CAD build for the part. Positions are in the model's coordinates, mm. A direction names the side the tool comes from. Give positions to 0.01 mm unless a question says otherwise; leave off trailing zeros. Write each loop counter-clockwise with the first axis right and the second up, starting at its lowest first coordinate (ties: lowest second). Pieces come first, ordered by that corner, then holes. Notation, with made-up numbers: (65, 12.5) - (85, 12.5) arc R22 cw to (85, 29.5) - close; hole circle Ø2 at (81.25, 88.5). An arc over 180 degrees is marked (long way). Answer as a JSON object with one key per item and string values.
from build123d import *
from build123d import SkipClean  # not in build123d's __all__

# Parameters (mm, degrees)
F1_DEPTH = 20
F0_W     = 2
F0_H     = 6.5
F5_DEPTH = 5
F6_DEPTH = 5


with BuildPart() as f1:
    # F0 (on Top) → F1 (new body, symmetric)
    with BuildSketch(Plane.XY):
        Polygon((-33.9359952807, -3.1263027601), (-33.9359952807, -23.1263027601), (-31.9359952807, -23.1263027601), (-32.4359952807, -6.1263027601), (-25.8359952807, -6.1263027601), (-25.8359952807, -23.1263027601), (-22.8359952807, -23.1263027601), (-17.8684814229, -20.8465269788), (-17.8684814229, -20.3465269788), (-17.8684814229, -13.8465269788), (-17.8684814229, -7.3465269788), (-17.8684814229, -6.8465269788), (-21.8359952807, -3.1263027601), align=None)
    extrude(amount=F1_DEPTH, both=True)

    # F0 (on Top) → F2 (revolve)
    with BuildSketch(Plane.XY):
        with Locations((-16.8684814229, -10.5965269788)):
            Rectangle(F0_W, F0_H)
    revolve(axis=Axis((-16.8684814229, -13.8465269788, 0), (1, 0, 0)))

    # F0 (on Top) → F3 (revolve)
    with BuildSketch(Plane.XY):
        Polygon((-9.0739962115, -8.8465269788), (-15.8684814229, -7.3465269788), (-15.8684814229, -13.8465269788), (-9.0739962115, -13.8465269788), align=None)
    revolve(axis=Axis((-4.8684814229, -13.8465269788, 0), (1, 0, 0)))

    # F0 (on Top) → F4 (revolve)
    with BuildSketch(Plane.XY):
        with BuildLine():
            Line((6.1315185771, -8.8465269788), (-9.0739962115, -8.8465269788))
            Line((-9.0739962115, -8.8465269788), (-9.0739962115, -13.8465269788))
            Line((-9.0739962115, -13.8465269788), (1.1315185771, -13.8465269788))
            ThreePointArc((1.1315185771, -13.8465269788), (2.5959846712, -10.3109930728), (6.1315185771, -8.8465269788))
        make_face()
        with BuildLine():
            Line((6.1315185771, -12.0965269788), (6.1315185771, -8.8465269788))
            ThreePointArc((6.1315185771, -8.8465269788), (2.5959846712, -10.3109930728), (1.1315185771, -13.8465269788))
            Line((1.1315185771, -13.8465269788), (4.3815185771, -13.8465269788))
            ThreePointArc((4.3815185771, -13.8465269788), (4.89408171, -12.6090901117), (6.1315185771, -12.0965269788))
        make_face()
        with BuildLine():
            Line((6.1315185771, -13.8465269788), (6.1315185771, -12.0965269788))
            ThreePointArc((6.1315185771, -12.0965269788), (4.89408171, -12.6090901117), (4.3815185771, -13.8465269788))
            Line((4.3815185771, -13.8465269788), (6.1315185771, -13.8465269788))
        make_face()
    revolve(axis=Axis((-4.8684814229, -13.8465269788, 0), (1, 0, 0)))

    # F0 (on Top) → F5 (cut, symmetric)
    with BuildSketch(Plane.XY):
        with BuildLine():
            Line((6.1315185771, -13.8465269788), (4.3815185771, -13.8465269788))
            ThreePointArc((4.3815185771, -13.8465269788), (4.89408171, -15.0839638459), (6.1315185771, -15.5965269788))
            Line((6.1315185771, -15.5965269788), (6.1315185771, -13.8465269788))
        make_face()
        with BuildLine():
            ThreePointArc((7.8815185771, -13.8465269788), (7.3689554442, -12.6090901117), (6.1315185771, -12.0965269788))
            Line((6.1315185771, -12.0965269788), (6.1315185771, -13.8465269788))
            Line((6.1315185771, -13.8465269788), (6.1315185771, -15.5965269788))
            ThreePointArc((6.1315185771, -15.5965269788), (7.3689554442, -15.0839638459), (7.8815185771, -13.8465269788))
        make_face()
        with BuildLine():
            Line((6.1315185771, -13.8465269788), (6.1315185771, -12.0965269788))
            ThreePointArc((6.1315185771, -12.0965269788), (4.89408171, -12.6090901117), (4.3815185771, -13.8465269788))
            Line((4.3815185771, -13.8465269788), (6.1315185771, -13.8465269788))
        make_face()
    extrude(amount=F5_DEPTH, both=True, mode=Mode.SUBTRACT)

    # F0 (on Top) → F6 (join, symmetric)
    with BuildSketch(Plane.XY):
        with BuildLine():
            Line((6.1315185771, -12.0965269788), (6.1315185771, -8.8465269788))
            ThreePointArc((6.1315185771, -8.8465269788), (2.5959846712, -10.3109930728), (1.1315185771, -13.8465269788))
            Line((1.1315185771, -13.8465269788), (4.3815185771, -13.8465269788))
            ThreePointArc((4.3815185771, -13.8465269788), (4.89408171, -12.6090901117), (6.1315185771, -12.0965269788))
        make_face()
        with BuildLine():
            Line((4.3815185771, -13.8465269788), (1.1315185771, -13.8465269788))
            ThreePointArc((1.1315185771, -13.8465269788), (2.5959846712, -17.3820608847), (6.1315185771, -18.8465269788))
            Line((6.1315185771, -18.8465269788), (6.1315185771, -15.5965269788))
            ThreePointArc((6.1315185771, -15.5965269788), (4.89408171, -15.0839638459), (4.3815185771, -13.8465269788))
        make_face()
        with BuildLine():
            ThreePointArc((11.1315185771, -13.8465269788), (9.667052483, -10.3109930728), (6.1315185771, -8.8465269788))
            Line((6.1315185771, -8.8465269788), (6.1315185771, -12.0965269788))
            ThreePointArc((6.1315185771, -12.0965269788), (7.3689554442, -12.6090901117), (7.8815185771, -13.8465269788))
            ThreePointArc((7.8815185771, -13.8465269788), (7.3689554442, -15.0839638459), (6.1315185771, -15.5965269788))
            Line((6.1315185771, -15.5965269788), (6.1315185771, -18.8465269788))
            ThreePointArc((6.1315185771, -18.8465269788), (9.667052483, -17.3820608847), (11.1315185771, -13.8465269788))
        make_face()
    with SkipClean():  # cleaning this boolean's faces spoils the solid; the shape is the same uncleaned
        extrude(amount=F6_DEPTH, both=True)


solid = f1.part
Item 1: Probe line 1 (X direction, y = -14, z = -0.5); line 2 (Y direction, x = -26, z = -8); line 3 (X direction, y = -19.25, z = 12). List the from-to ranges inside material, lowest first. Write a range as from..to.
Entries:
{"line 1": "-33.94..-32.2, -25.84..4.39, 7.87..11.13", "line 2": "-6.13..-3.13", "line 3": "-33.94..-32.05, -25.84..-17.87"}
Item 2: Which spindle directions (+Z, -Z, +X, -X, +Y, -Y) get a long thin tool onto all of the face, cutting with end or side? Do faces 1 (the flat face through (-25.836, -15, 0)), 2 (the flat face through (8.3, -13.8, 5)), 3 (the cylindrical face through (-3.267, -14.497, 4.957)), 4 (the flat face through (8.3, -13.8, -5)). Say none if no direction does.
Entries:
{"face 1": "+Z, -Z, -Y", "face 2": "+Z, +X, +Y, -Y", "face 3": "none", "face 4": "-Z, +X, +Y, -Y"}
Item 3: Flat gauge pins, fed straight in: P1, Ø4, axis at y = -15.5, z = -6.5, coming from the +X side; P2, Ø3, axis at y = -20.5, z = 7.5, coming from the +X side; P3, Ø3, axis at x = -2.5, y = -17.5, coming from the +Z side. Where does each tip first touch, or does it go through?
Entries:
{"P1": "x = 11.12", "P2": "x = -17.87", "P3": "z = 4.51"}
Item 4: Cut at C-C (y = -14.5). State how many separate pieces and enclosed holes the cut face has, and give its area (3 significant figures).
Entries:
{"separate pieces": "3", "enclosed holes": "0", "area": "660 mm2"}
Item 5: Cut at D-D (x = -20.5). Give the cut face in (y, z).
Entries:
{"outline": "(-22.05, -20) - (-4.38, -20) - (-4.38, 20) - (-22.05, 20) - close"}
Item 6: Cut at A-A (z = -11.5). Give the cut face in (x, y).
Entries:
{"outline": "(-33.94, -23.13) - (-31.94, -23.13) - (-32.44, -6.13) - (-25.84, -6.13) - (-25.84, -23.13) - (-22.84, -23.13) - (-17.87, -20.85) - (-17.87, -6.85) - (-21.84, -3.13) - (-33.94, -3.13) - close"}
Item 7: Cut at B-B (x = -4.5). Give the cut face in (y, z), and give its area (3 significant figures).
Entries:
{"outline": "circle Ø10 at (-13.85, 0)", "area": "78.5 mm2"}
